Check sheet for the drawn part. Datum: minimum x, y, z corner. Units: mm. Round coordinates to 2 decimals unless told otherwise and drop trailing zeros. Write each loop counter-clockwise with the first axis right and the second up, starting at its lowest first coordinate (ties: lowest second). Pieces come first, ordered by that corner, then holes.
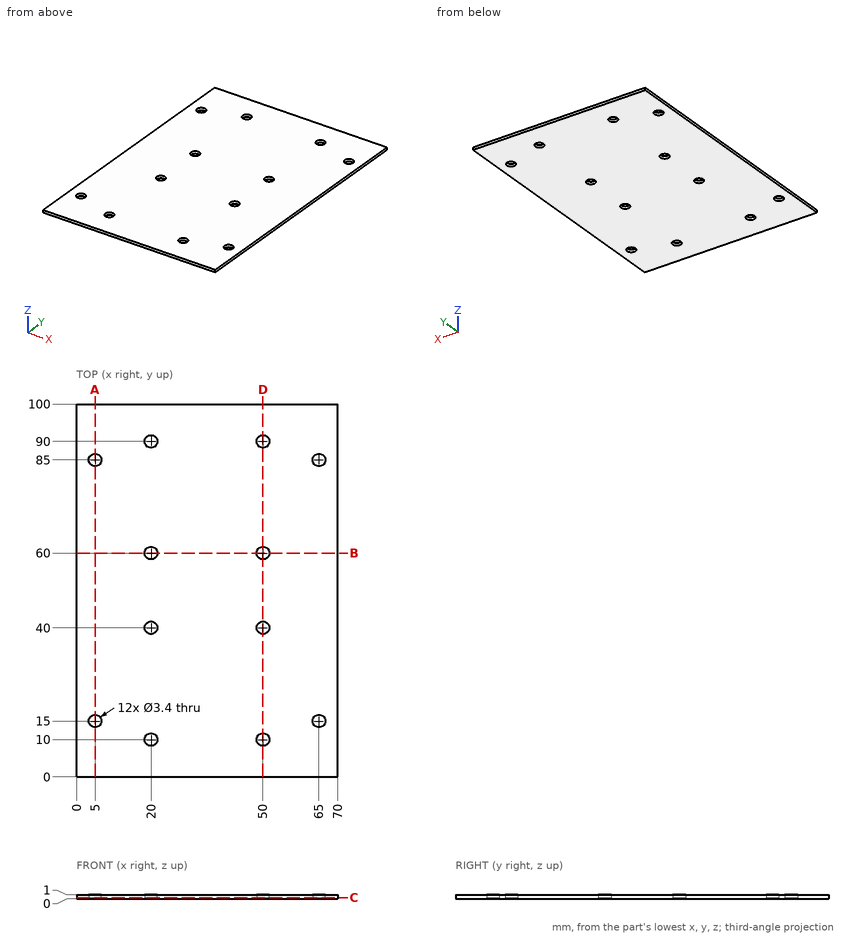
Q1. Sectioned sample at C-C (z = 0.3). Give the number of separate pieces and of enclosed holes in the cut face, plus the area to 3 significant figures.
Recorded:
separate pieces: 1
enclosed holes: 12
area: 6,890 mm2
Q2. Sectioned sample at A-A (x = 5). Enter the section's corners in (y, z).
Recorded:
outline: (0, 0) - (13.3, 0) - (13.3, 1) - (0, 1) - close; (16.7, 0) - (83.3, 0) - (83.3, 1) - (16.7, 1) - close; (86.7, 0) - (100, 0) - (100, 1) - (86.7, 1) - close
Q3. Sectioned sample at D-D (x = 50). Enter the section's corners in (y, z).
Recorded:
outline: (0, 0) - (8.3, 0) - (8.3, 1) - (0, 1) - close; (11.7, 0) - (38.3, 0) - (38.3, 1) - (11.7, 1) - close; (41.7, 0) - (58.3, 0) - (58.3, 1) - (41.7, 1) - close; (61.7, 0) - (88.3, 0) - (88.3, 1) - (61.7, 1) - close; (91.7, 0) - (100, 0) - (100, 1) - (91.7, 1) - close
Q4. Material ranges on line 1 along Y through (x, z) = (20, 0.4); line 2 along X through (y, z) = (10, 0.65); line 3 along X through (y, z) = (15, 0.8), recorded low to high.
Recorded:
line 1: y = 0 to 8.3, 11.7 to 38.3, 41.7 to 58.3, 61.7 to 88.3, 91.7 to 100
line 2: x = 0 to 18.3, 21.7 to 48.3, 51.7 to 70
line 3: x = 0 to 3.3, 6.7 to 63.3, 66.7 to 70
Q5. Sectioned sample at B-B (y = 60). Enter the section's corners in (x, z).
Recorded:
outline: (0, 0) - (18.3, 0) - (18.3, 1) - (0, 1) - close; (21.7, 0) - (48.3, 0) - (48.3, 1) - (21.7, 1) - close; (51.7, 0) - (70, 0) - (70, 1) - (51.7, 1) - close
